Build history of the part. All positions in model axes, mm. A direction names the side the tool comes from. Round coordinates to 2 decimals unless told otherwise and drop trailing zeros. Loops run counter-clockwise (first coordinate to the right, second up) from the corner with the lowest first, then second, coordinate; pieces in that order, holes last. Notation, with made-up numbers: (23, 76) -> (78, 76) arc R9 cw to (78, 85) -> close; hole circle Ø3 at (13, 89). An arc over 180 degrees is marked (long way). Put each result on its own line as item: value. Start each with the question number.
Item 1: Drill centre lines: probe 1 along Y at (x, z) = (94, -20); probe 2 along Y at (x, z) = (102.5, -10); probe 3 along Y at (x, z) = (7, -12.5). Where is each one in solid material? Low to high. Write a range as [from, to].
Item 2: Flat gauge pins, fed straight in: pin 1 Ø6 at (x, z) = (96.5, -30) entering from -Y; pin 2 Ø10 at (y, z) = (-22.63, 22.63) entering from -X; pin 3 Ø24 at (y, z) = (-14, 3.5) entering from -X; pin 4 Ø6.5 at (x, z) = (6.5, -11) entering from -Y. Where does each tip first touch, or does it go through?
Item 3: Pull direction Z, two halves, no side cores. Call faces 4 (the cylindrical face through (61.8, -7.2, 34.5)), 5 (the flat face through (114, -9, -26)), 6 (the cylindrical face through (8.619, -17.085, -18.251)), 7 (the cylindrical face through (103.446, -11.157, 34.844)): +Z half, -Z half, draft (parallel to the pull), parting line (faces both ways), or undercut.
Item 4: Cut at B-B, the plane x = 124.5. List the corners of the cut face in (y, z), plus the area to 3 significant figures.
Item 5: Tool access for faces 1 (the flat face through (5, -4, 8)), 2 (the flat face through (51, 0, 16)), 3 (the cylindrical face through (112, -15, 12)): list every direction of +Z, -Z, +X, -X, +Y, -Y with a clear straight run to the whole face (end or side of a thin tool).
Item 6: Cut at A-A, the plane x = 31.5. Count the separate pieces of the cut face and the enclosed holes in it, plus the area to 3 significant figures.
```python
from build123d import *

# Parameters (mm, degrees)
ZAOKR_GLENIE1_R            = 2
WYTNIJ_WYCI_GNI_CIE1_DEPTH = 134
SZKIC4_R                   = 3.75
WYTNIJ_WYCI_GNI_CIE2_DEPTH = 115
SZYK_KO_OWY1_COUNT         = 9
SZYK_KO_OWY1_ANGLE         = 240
WYTNIJ_WYCI_GNI_CIE3_DEPTH = 41
WYTNIJ_WYCI_GNI_CIE4_DEPTH = 10
ZAOKR_GLENIE2_R            = 1
ZAOKR_GLENIE3_R            = 1


with BuildPart() as part:
    # Szkic2 → Obrót1 (revolve)
    with BuildSketch(Plane.XY):
        Polygon((0, 0), (0, 25), (19, 25), (19, 40), (47.5, 40), (50, 37.5), (83, 37.5), (85.5, 40), (114, 40), (114, 25), (133, 25), (133, 0), align=None)
    revolve(axis=Axis((133, 0, 0), (-1, 0, 0)))

    # Zaokrąglenie1
    zaokr_glenie1_edges = [part.edges().sort_by_distance(p)[0] for p in [
        (114, -25, 0),
        (19, -25, 0),
    ]]
    fillet(zaokr_glenie1_edges, radius=ZAOKR_GLENIE1_R)

    # Szkic3 → Wytnij-wyciągnięcie1 (cut, through all)
    with BuildSketch(Plane.ZY):
        with BuildLine():
            Line((0, 0), (0, 7))
            Line((0, 7), (-12, 7))
            ThreePointArc((-12, 7), (-15, 10), (-12, 13))
            Line((-12, 13), (0, 13))
            Line((0, 13), (0, 40))
            ThreePointArc((0, 40), (28.284271247, 28.284271247), (40, 0))
            Line((40, 0), (0, 0))
        make_face()
    extrude(amount=-WYTNIJ_WYCI_GNI_CIE1_DEPTH, mode=Mode.SUBTRACT)

    # Szkic4 → Wytnij-wyciągnięcie2 (cut, through all)
    with BuildSketch(Plane.ZY.offset(-19)):
        with Locations((-8.282209443, 30.909626441)):
            Circle(SZKIC4_R)
    wytnij_wyci_gni_cie2 = extrude(amount=-WYTNIJ_WYCI_GNI_CIE2_DEPTH, mode=Mode.SUBTRACT)

    # Szyk kołowy1: Wytnij-wyciągnięcie2 ×9 about axis
    szyk_ko_owy1_axis = Axis((0, 0, 0), (-1, 0, 0))
    for i in range(1, SZYK_KO_OWY1_COUNT):
        add(wytnij_wyci_gni_cie2.rotate(szyk_ko_owy1_axis, i * SZYK_KO_OWY1_ANGLE / (SZYK_KO_OWY1_COUNT - 1)), mode=Mode.SUBTRACT)

    # Szkic5 → Wytnij-wyciągnięcie3 (cut, through all)
    with BuildSketch(Plane(origin=(0, 0, 0), x_dir=(1, 0, 0), z_dir=(0, 1, 0))):
        with BuildLine():
            Line((101.279227454, -25.208360839), (105.810766389, -27.321452148))
            ThreePointArc((105.810766389, -27.321452148), (151.26284287, -63.800600209), (127.79055467, -10.45576741))
            Line((127.79055467, -10.45576741), (126.922313782, -5.531728645))
            ThreePointArc((126.922313782, -5.531728645), (111.693349985, -12.23263309), (101.279227454, -25.208360839))
        make_face()
    extrude(amount=-WYTNIJ_WYCI_GNI_CIE3_DEPTH, mode=Mode.SUBTRACT)

    # Szkic6 → Wytnij-wyciągnięcie4 (cut)
    with BuildSketch(Plane.ZY):
        with BuildLine():
            Line((-19.899748742, 3), (-5, 3))
            ThreePointArc((-5, 3), (-4.292893219, 2.707106781), (-4, 2))
            Line((-4, 2), (-4, -3))
            ThreePointArc((-4, -3), (-3.707106781, -3.707106781), (-3, -4))
            Line((-3, -4), (19.364916731, -4))
            ThreePointArc((19.364916731, -4), (20.155486146, -4.387627564), (20.333162568, -5.25))
            ThreePointArc((20.333162568, -5.25), (-3.685711089, -20.674030419), (-20.894736179, 2.1))
            ThreePointArc((-20.894736179, 2.1), (-20.570569135, 2.741619849), (-19.899748742, 3))
        make_face()
    extrude(amount=-WYTNIJ_WYCI_GNI_CIE4_DEPTH, mode=Mode.SUBTRACT)

    # Zaokrąglenie2
    zaokr_glenie2_edges = [part.edges().sort_by_distance(p)[0] for p in [
        (10, -4.387627564, 20.155486146),
        (10, -20.674030419, -3.685711089),
        (10, 2.741619849, -20.570569135),
        (10, 3, -12.449874371),
        (10, 2.707106781, -4.292893219),
        (10, -0.5, -4),
        (10, -3.707106781, -3.707106781),
        (10, -4, 8.182458366),
    ]]
    fillet(zaokr_glenie2_edges, radius=ZAOKR_GLENIE2_R)

    # Zaokrąglenie3
    zaokr_glenie3_edges = [part.edges().sort_by_distance(p)[0] for p in [
        (0, -4.387627564, 20.155486146),
        (0, -20.674030419, -3.685711089),
        (0, 2.741619849, -20.570569135),
        (0, 3, -12.449874371),
        (0, 2.707106781, -4.292893219),
        (0, -0.5, -4),
        (0, -3.707106781, -3.707106781),
        (0, -4, 8.182458366),
    ]]
    fillet(zaokr_glenie3_edges, radius=ZAOKR_GLENIE3_R)


solid = part.part
```
Reply:
1. probe 1: y = [-34.64, -25.3], [-19.95, 19.95], [25.3, 34.64]
1. probe 2: y = [-38.73, -34.24], [-27.58, 7], [13, 27.58], [34.24, 38.73]
1. probe 3: y = [-21.65, -16.87], [3, 7.04], [12.96, 21.65]
2. pin 1: stops at y = -29.51
2. pin 2: stops at x = 19
2. pin 3: stops at x = 0
2. pin 4: stops at y = -23.77
3. face 4: undercut
3. face 5: draft
3. face 6: parting line
3. face 7: +Z half
4. outline: (-24.26, 6.05) arc R25 ccw (long way) to (25, 0) -> (13, 0) -> (13, -12) arc R3 cw to (7, -12) -> (7, 0) -> (0, 0) -> (0, 6.05) -> close
4. area: 1,050 mm^2
5. face 1: -X
5. face 2: +Z, +X, -X, +Y
5. face 3: +Y, -Y
6. separate pieces: 1
6. enclosed holes: 9
6. area: 3,290 mm^2
